```python
from build123d import *

# Parameters (mm, degrees)
CUT_EXTRUDE1_DEPTH      = 32.590851198
CUT_EXTRUDE1_DEPTH_BACK = 32.590851198
SKETCH2_R               = 2.1828125


with BuildPart() as part:
    # Sketch1 → Revolve1 (revolve)
    with BuildSketch(Plane.XY, mode=Mode.PRIVATE) as revolve1_sk:
        with BuildLine():
            Line((0, 0), (20.6375, 0))
            ThreePointArc((20.6375, 0), (21.760032015, 0.464967985), (22.225, 1.5875))
            Line((22.225, 1.5875), (22.225, 3.175))
            Line((22.225, 3.175), (0, 3.175))
            Line((0, 3.175), (0, 0))
        make_face()
    revolve(revolve1_sk.sketch.rotate(Axis((0, 0, 0), (0, 1, 0)), 90), axis=Axis((0, 0, 0), (0, 1, 0)))

    # Sketch2 → Cut-Extrude1 (cut, two sides: drawn at the far end of the back side and taken through both)
    with BuildSketch(Plane(origin=(0, 3.175, 0), x_dir=(1, 0, 0), z_dir=(0, 1, 0)).offset(-CUT_EXTRUDE1_DEPTH_BACK)):
        with Locations(Location((0, 0, 0), (0, 0, 270))):
            Circle(SKETCH2_R)
        with Locations(Location((12.7, 0, 0), (0, 0, 270))):
            Circle(SKETCH2_R)
        with Locations(Location((-12.7, 0, 0), (0, 0, 270))):
            Circle(SKETCH2_R)
    extrude(amount=CUT_EXTRUDE1_DEPTH + CUT_EXTRUDE1_DEPTH_BACK, mode=Mode.SUBTRACT)


solid = part.part
```
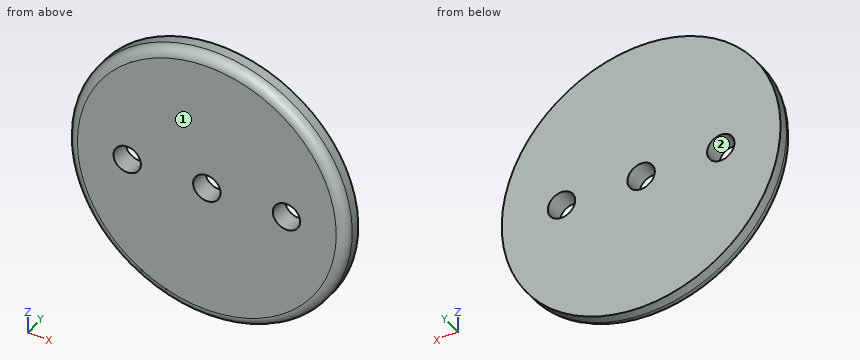
Source: CAD feature listing. Evaluate the final solid. Frame: model axes, mm. Face numbers are marked on the shaded views. Round coordinates to 2 decimals unless told otherwise and drop trailing zeros. Write each loop counter-clockwise with the first axis right and the second up, starting at its lowest first coordinate (ties: lowest second). Pieces come first, ordered by that corner, then holes. Notation, with made-up numbers: M 68,73 L 80,73 A16 ccw 80,86 Z; hole C -28.5,35.5 d9. An arc over 180 degrees is marked long. Answer as a JSON object with one key per item and string values. Group by question number.
(1) Section query B-B on z = 0. Output: boundary loops of the cut face in (x, y) (1 decimal).
(2) Mould query, pull axis Z, two halves, no side actions, for the marked faces 1 and 2. Classes: +Z half, -Z half, draft (parallel to the pull), parting line (faces both ways), or undercut.
(3) Section query A-A on x = 0. Output: boundary loops of the cut face in (y, z) (1 decimal), then the cut area to 3 significant figures.
(4) First-contact query: pin 1 (3.5 mm diameter, centred on x = 0, z = 0, fed in from +Y); pin 2 (1 mm diameter, centred on y = 2.5, z = 11.5, fed in from +X). Flat tips, straight axial feed; report the tip coordinate or a pass-through.
(5) Section query C-C on y = 2.35. Output: boundary loops of the cut face in (x, z) (3 decimals).
(6) Ray query, line 1 (X direction, y = 1.9, z = 0) (3 decimals); line 2 (X direction, y = 2.7, z = -1); line 3 (Y direction, x = 10.5, z = -18) (3 decimals). Return the intervals inside material, ascending. Write a range as [from, to].
Computed values:
{
 "1": {"outline": "M -22.2,1.6 A1.6 ccw -20.6,0 L -14.9,0 L -14.9,3.2 L -22.2,3.2 Z; M -10.5,0 L -2.2,0 L -2.2,3.2 L -10.5,3.2 Z; M 2.2,0 L 10.5,0 L 10.5,3.2 L 2.2,3.2 Z; M 14.9,0 L 20.6,0 A1.6 ccw 22.2,1.6 L 22.2,3.2 L 14.9,3.2 Z"},
 "2": {"face 1": "draft", "face 2": "undercut"},
 "3": {"outline": "M 0,-20.6 A1.6 ccw 1.6,-22.2 L 3.2,-22.2 L 3.2,-2.2 L 0,-2.2 Z; M 0,2.2 L 3.2,2.2 L 3.2,22.2 L 1.6,22.2 A1.6 ccw 0,20.6 Z", "area": "126 mm^2"},
 "4": {"pin 1": "through", "pin 2": "x = 19.31"},
 "5": {"outline": "C 0,0 d44.45; hole C -12.7,0 d4.366; hole C 0,0 d4.366; hole C 12.7,0 d4.366"},
 "6": {"line 1": "[-22.225, -14.883], [-10.517, -2.183], [2.183, 10.517], [14.883, 22.225]", "line 2": "[-22.2, -14.64], [-10.76, -1.94], [1.94, 10.76], [14.64, 22.2]", "line 3": "[0.013, 3.175]"}
}
